```python
from build123d import *

# Parameters (mm, degrees)
F0_W     = 35
F0_H     = 16
F1_DEPTH = 18
F2_R     = 8
F3_DEPTH = 40
F4_W     = 4
F4_H     = 3
F5_DEPTH = 25
F6_R     = 1.5
F7_DEPTH = 18.001


with BuildPart() as f1:
    # F0 (on Top) → F1 (new body)
    with BuildSketch(Plane.XY):
        Rectangle(F0_W, F0_H)
    extrude(amount=F1_DEPTH)

    # F2 (on face) → F3 (cut)
    with BuildSketch(Plane(origin=(-17.5, 0, 0), x_dir=(0, -1, 0), z_dir=(-1, 0, 0))):
        with Locations((0, 18)):
            Circle(F2_R)
    extrude(amount=-F3_DEPTH, mode=Mode.SUBTRACT)

    # F4 (on face) → F5 (cut)
    with BuildSketch(Plane.XZ.offset(8)):
        with Locations((-11.5, 6.5)):
            Rectangle(F4_W, F4_H)
        with Locations((11.5, 6.5)):
            Rectangle(F4_W, F4_H)
    extrude(amount=-F5_DEPTH, mode=Mode.SUBTRACT)

    # F6 (on face) → F7 (cut, through all)
    with BuildSketch(Plane(origin=(0, 0, 0), x_dir=(1, 0, 0), z_dir=(0, 0, -1))):
        Circle(F6_R)
    extrude(amount=-F7_DEPTH, mode=Mode.SUBTRACT)

    # F8 (on Right) → F9 (revolve, cut)
    with BuildSketch(Plane.YZ):
        Polygon((-4.5, 11.5), (0, 6), (0, 11.5), align=None)
    revolve(axis=Axis((0, 0, 8.75), (0, 0, -1)), mode=Mode.SUBTRACT)


solid = f1.part
```
Design review of the part built by this model. Coordinates are the model's own, in mm. A direction names the side the tool comes from. Give positions to 0.01 mm unless a question says otherwise; leave off trailing zeros. Order: outer loops, then holes, each group sorted by start corner. A loop starts at its lowest first (then second) coordinate and runs counter-clockwise, first axis right, second up. Notation, with made-up numbers: (77.25, 0) -> (81.25, 0) arc R22 cw to (81.25, 17) -> close; hole circle Ø6 at (-6.5, 42). An arc over 180 degrees is marked (long way). Write each question's results on one line, items separated by ' | '. Start each with the question number.
Q1. Add section C-C on z = 13.25. Give the boundary of the cut face in (x, y).
Q2. Add section A-A on x = 0. Give the boundary of the cut face in (y, z).
Q3. Add section B-B on y = 0. Give the boundary of the cut face in (x, z).
Q4. Add section D-D on y = 5.75. Give the boundary of the cut face in (x, z), and give its area (3 significant figures).
Q5. For pin 1 (4 mm diameter, centred on x = 10.5, y = 2.5, fed in from +Z); pin 2 (3 mm diameter, centred on x = 10.5, y = 0, fed in from +Z); pin 3 (4 mm diameter, centred on x = 0, y = 0, fed in from +Z), all flat-tipped, find the tip position at first contact; note any pin that passes through.
Q6. Machinability: for faces 1 (the cylindrical face through (-0.325, 1.464, 3.862)), 2 (the flat face through (-9.5, 0, 6)), which of the approach directions +Z, -Z, +X, -X, +Y, -Y give a long, thin tool a straight path to every point of the face, cutting with its end or side? Answer none if there is none.
Q7. Wall thickness on L1, parallel to X at y = -6.75, z = 7.5; L2, parallel to X at y = 0, z = 6; L3, parallel to Y at x = 0, z = 2.25: over which ranges is each line inside the solid? List them lowest first. Write a range as from..to.
Q8. Mouldability with a two-part tool opening along Y and no side actions: class faces 3 (the flat face through (0, -8, 9)), 4 (the conical face through (-0.072, 1.635, 8)), 5 (the flat face through (-12, 0, 5)) as +Y half, -Y half, draft (parallel to the pull), parting line (faces both ways), or undercut.
Found:
1) outline: (-17.5, -8) -> (17.5, -8) -> (17.5, -6.44) -> (-17.5, -6.44) -> close; (-17.5, 6.44) -> (17.5, 6.44) -> (17.5, 8) -> (-17.5, 8) -> close
2) outline: (-8, 0) -> (-1.5, 0) -> (-1.5, 7.83) -> (-4.3, 11.25) arc R8 cw to (-8, 18) -> close; (1.5, 0) -> (8, 0) -> (8, 18) arc R8 cw to (4.3, 11.25) -> (1.5, 7.83) -> close
3) outline: (-17.5, 0) -> (-1.5, 0) -> (-1.5, 7.83) -> (-3.27, 10) -> (-17.5, 10) -> close; (1.5, 0) -> (17.5, 0) -> (17.5, 10) -> (3.27, 10) -> (1.5, 7.83) -> close; hole (-13.5, 5) -> (-9.5, 5) -> (-9.5, 8) -> (-13.5, 8) -> close; hole (9.5, 5) -> (13.5, 5) -> (13.5, 8) -> (9.5, 8) -> close
4) outline: (-17.5, 0) -> (17.5, 0) -> (17.5, 12.44) -> (-17.5, 12.44) -> close; hole (-13.5, 5) -> (-9.5, 5) -> (-9.5, 8) -> (-13.5, 8) -> close; hole (9.5, 5) -> (13.5, 5) -> (13.5, 8) -> (9.5, 8) -> close | area: 411 mm2
5) pin 1: stops at z = 11.39 | pin 2: stops at z = 10.14 | pin 3: stops at z = 8.44
6) face 1: +Z, -Z | face 2: +Y, -Y
7) L1: x = -17.5..-13.5, -9.5..9.5, 13.5..17.5 | L2: x = -17.5..-13.5, -9.5..-1.5, 1.5..9.5, 13.5..17.5 | L3: y = -8..-1.5, 1.5..8
8) face 3: -Y half | face 4: undercut | face 5: draft
